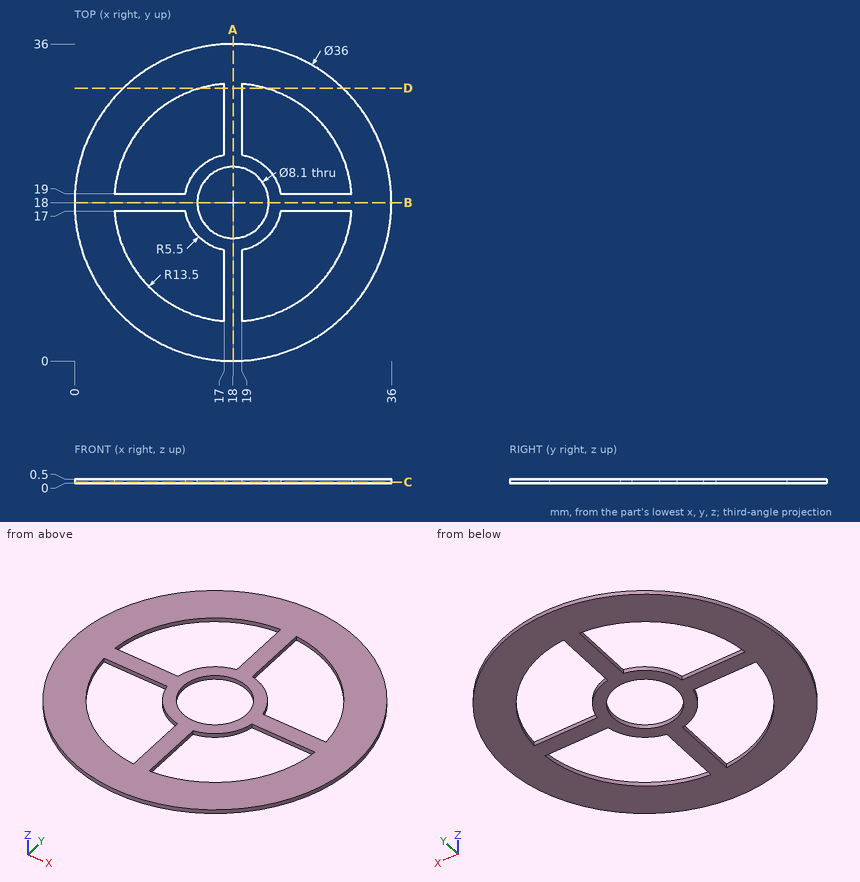
Could you check a few things on this drawing? It's one solid part, dimensions in mm from its lowest x, y, z. Give positions to 0.01 mm unless a question says otherwise; leave off trailing zeros. Order: outer loops, then holes, each group sorted by start corner. A loop starts at its lowest first (then second) coordinate and runs counter-clockwise, first axis right, second up. Notation, with made-up numbers: (57, -38) - (63, -38) arc R14 ccw to (63, -12) - close; hole circle Ø3 at (-5, 74). An arc over 180 degrees is marked (long way). One line per question, with ' | ' between items. Start each with the question number.
Item 1: I need wall thicknesses on probe 1 along Y at (x, z) = (18, 0.35); probe 2 along X at (y, z) = (11, 0.25); probe 3 along X at (y, z) = (24.5, 0.45). Which ranges of each line are inside material? Lowest first, please. Write a range as [from, to].
Item 2: I want a section at A-A on x = 18. Write out the boundary of the cut face in (y, z), then the cut area to 4 significant figures.
Item 3: I want a section at C-C on z = 0.15. Write out the boundary of the cut face in (x, y).
Item 4: I want a section at D-D on y = 31. Write out the boundary of the cut face in (x, z).
Verdict:
1) probe 1: [0, 13.95], [22.05, 36] | probe 2: [1.42, 6.46], [17, 19], [29.54, 34.58] | probe 3: [1.21, 6.17], [17, 19], [29.83, 34.79]
2) outline: (0, 0) - (13.95, 0) - (13.95, 0.5) - (0, 0.5) - close; (22.05, 0) - (36, 0) - (36, 0.5) - (22.05, 0.5) - close | area: 13.95 mm^2
3) outline: circle Ø36 at (18, 18); hole (4.54, 17) arc R13.5 ccw to (17, 4.54) - (17, 12.59) arc R5.5 cw to (12.59, 17) - close; hole (4.54, 19) - (12.59, 19) arc R5.5 cw to (17, 23.41) - (17, 31.46) arc R13.5 ccw to start; hole circle Ø8.1 at (18, 18); hole (19, 4.54) arc R13.5 ccw to (31.46, 17) - (23.41, 17) arc R5.5 cw to (19, 12.59) - close; hole (19, 23.41) arc R5.5 cw to (23.41, 19) - (31.46, 19) arc R13.5 ccw to (19, 31.46) - close
4) outline: (5.55, 0) - (14.36, 0) - (14.36, 0.5) - (5.55, 0.5) - close; (17, 0) - (19, 0) - (19, 0.5) - (17, 0.5) - close; (21.64, 0) - (30.45, 0) - (30.45, 0.5) - (21.64, 0.5) - close
